Check sheet for the modelled part. Datum: model origin and axes. Units: mm. Face numbers are marked on the shaded views. A direction names the side the tool comes from. Round coordinates to 2 decimals unless told otherwise and drop trailing zeros. Order: outer loops, then holes, each group sorted by start corner. A loop starts at its lowest first (then second) coordinate and runs counter-clockwise, first axis right, second up.
```python
from build123d import *

# Parameters (mm, degrees)
SKETCH_2_R             = 11
SKETCH_2_R_2           = 1.5
EXTRUDE_483_DEPTH      = 4
SKETCH_3_W             = 18
SKETCH_3_H             = 26.8
EXTRUDE_726_DEPTH      = 4
EXTRUDE_922_DEPTH      = 2
SKETCH_5_R             = 1.5
CUT_EXTRUDE_1097_DEPTH = 51.175093423
SKETCH_7_W             = 18
SKETCH_7_H             = 22.8
CUT_EXTRUDE_1_DEPTH    = 1


with BuildPart() as part:
    # Эскиз2 → Extrude 483 (new body)
    with BuildSketch(Plane(origin=(0, 0, 0), x_dir=(1, 0, 0), z_dir=(0, 1, 0))):
        with BuildLine():
            Line((-15.5, -20.5), (15.5, -20.5))
            ThreePointArc((15.5, -20.5), (19.035533906, -19.035533906), (20.5, -15.5))
            Line((20.5, -15.5), (20.5, 15.5))
            ThreePointArc((20.5, 15.5), (19.035533906, 19.035533906), (15.5, 20.5))
            Line((15.5, 20.5), (-15.5, 20.5))
            ThreePointArc((-15.5, 20.5), (-19.035533906, 19.035533906), (-20.5, 15.5))
            Line((-20.5, 15.5), (-20.5, -15.5))
            ThreePointArc((-20.5, -15.5), (-19.035533906, -19.035533906), (-15.5, -20.5))
        make_face()
        with Locations(Location((0, 0, 0), (0, 0, 270))):
            Circle(SKETCH_2_R, mode=Mode.SUBTRACT)
        with Locations(Location((-15.5, 15.5, 0), (0, 0, 270))):
            Circle(SKETCH_2_R_2, mode=Mode.SUBTRACT)
        with Locations(Location((15.5, -15.5, 0), (0, 0, 90))):
            Circle(SKETCH_2_R_2, mode=Mode.SUBTRACT)
        with Locations(Location((-15.5, -15.5, 0), (0, 0, 90))):
            Circle(SKETCH_2_R_2, mode=Mode.SUBTRACT)
        with Locations(Location((15.5, 15.5, 0), (0, 0, 270))):
            Circle(SKETCH_2_R_2, mode=Mode.SUBTRACT)
    extrude(amount=EXTRUDE_483_DEPTH)

    # Эскиз3 → Extrude 726 (add)
    with BuildSketch(Plane.XY.offset(20.5)):
        with Locations((0, -9.4)):
            Rectangle(SKETCH_3_W, SKETCH_3_H)
    extrude_726 = extrude(amount=EXTRUDE_726_DEPTH)

    # Эскиз4 → Extrude 922 (add)
    with BuildSketch(Plane.XZ.offset(22.8)):
        with BuildLine():
            Line((9, 24.5), (-9, 24.5))
            Line((-9, 24.5), (-9, 32.5))
            ThreePointArc((-9, 32.5), (-7.242640687, 36.742640687), (-3, 38.5))
            Line((-3, 38.5), (3, 38.5))
            ThreePointArc((3, 38.5), (7.242640687, 36.742640687), (9, 32.5))
            Line((9, 32.5), (9, 24.5))
        make_face()
    extrude_922 = extrude(amount=-EXTRUDE_922_DEPTH)

    # Эскиз5 → Cut-Extrude 1097 (cut, through all)
    with BuildSketch(Plane(origin=(0, -20.8, 0), x_dir=(1, 0, 0), z_dir=(0, 1, 0))):
        with Locations(Location((0, -29.678729535, 0), (0, 0, 270))):
            Circle(SKETCH_5_R)
    cut_extrude_1097 = extrude(amount=-CUT_EXTRUDE_1097_DEPTH, mode=Mode.SUBTRACT)

    # Эскиз7 → Вырез-Вытянуть1 (cut)
    with BuildSketch(Plane(origin=(0, 0, 20.5), x_dir=(-1, 0, 0), z_dir=(0, 0, -1))):
        with Locations((0, -11.4)):
            Rectangle(SKETCH_7_W, SKETCH_7_H)
    cut_extrude_1 = extrude(amount=-CUT_EXTRUDE_1_DEPTH, mode=Mode.SUBTRACT)

    # Зеркальное отражение1: Extrude 726, Extrude 922, Cut-Extrude 1097, Вырез-Вытянуть1 across plane
    add(extrude_726.mirror(Plane.XY))
    add(extrude_922.mirror(Plane.XY))
    add(cut_extrude_1097.mirror(Plane.XY), mode=Mode.SUBTRACT)
    add(cut_extrude_1.mirror(Plane.XY), mode=Mode.SUBTRACT)


solid = part.part
```
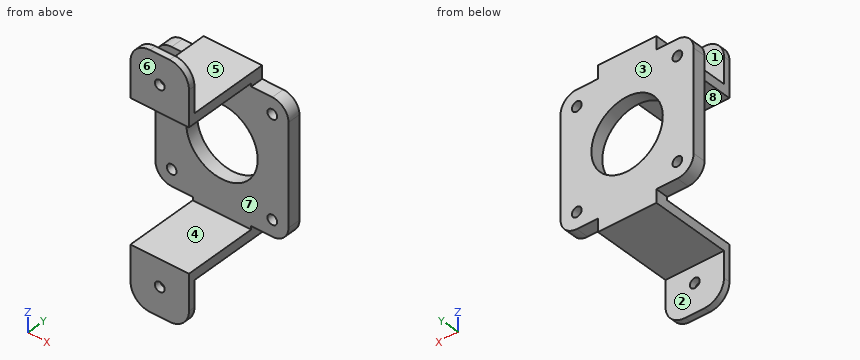
Item 1: Release check for a two-part mould opening along Z. For the marked faces 5, 6, 7 and 8 record: released by +Z, released by -Z, zero draft, split by the parting line, or undercut.
Answer:
face 5: released by +Z
face 6: zero draft
face 7: undercut
face 8: undercut
Item 2: Access from +Z, -Z, +X, -X, +Y, -Y to the whole of each face (thin tool, end or side, straight path). Record for the marked faces 1, 2, 3 and 4.
Answer:
face 1: +Z, +X, -X, +Y
face 2: -Z, +X, -X, +Y
face 3: +Z, -Z, +X, -X, +Y
face 4: +X, -X, -Y
Item 3: Sectioned sample at D-D (z = 23). Record the cut outline in (x, y), and give its area (3 significant figures).
Answer:
outline: (-9, -22.8) - (9, -22.8) - (9, 4) - (-9, 4) - close
area: 482 mm2
Item 4: Sectioned sample at C-C (x = -5.5). Record the cut outline in (y, z), and give its area (3 significant figures).
Answer:
outline: (-22.8, -37.95) - (-20.8, -37.95) - (-20.8, -24.5) - (4, -24.5) - (4, -9.53) - (0, -9.53) - (0, -21.5) - (-22.8, -21.5) - close; (-22.8, 21.5) - (0, 21.5) - (0, 9.53) - (4, 9.53) - (4, 24.5) - (-20.8, 24.5) - (-20.8, 37.95) - (-22.8, 37.95) - close
area: 310 mm2
Item 5: Sectioned sample at A-A (y = -15.25). Record the cut outline in (x, z).
Answer:
outline: (-9, -24.5) - (9, -24.5) - (9, -21.5) - (-9, -21.5) - close; (-9, 21.5) - (9, 21.5) - (9, 24.5) - (-9, 24.5) - close
Item 6: Go/stop test with flat-tipped pins: P1, Ø5.5, axis at x = -3.5, y = -3.5, coming from the +Z side; P2, Ø1.5, axis at x = 8.5, z = -30, coming from the +Y side; P3, Ø2.5, axis at x = 0, z = 29.68, coming from the -Y side; P4, Ø1.2, axis at x = 11, y = 1.5, coming from the +Z side. Record where each tip stops, or that it passes through.
Answer:
P1: stops at z = 24.5
P2: stops at y = -20.8
P3: passes through
P4: stops at z = 20.5
Item 7: Scan lines: line 1 along Z through (x, y) = (0, -2); line 2 along X through (y, z) = (1.8, -15.5); line 3 along Z through (x, y) = (-15, 2). Record each from-to range of solid material in increasing order.
Answer:
line 1: z = -24.5 to -21.5, 21.5 to 24.5
line 2: x = -20.5 to -17, -14 to 14, 17 to 20.5
line 3: z = -20.5 to -16.91, -14.09 to 14.09, 16.91 to 20.5
Item 8: Sectioned sample at B-B (z = 0). Record the cut outline in (x, y), and give its area (3 significant figures).
Answer:
outline: (-20.5, 0) - (-11, 0) - (-11, 4) - (-20.5, 4) - close; (11, 0) - (20.5, 0) - (20.5, 4) - (11, 4) - close
area: 76.0 mm2
